Autodesk Inventor part; units mm, degrees
ref_plane "YZ Plane" through (0, 0, 0) normal (1, 0, 0) x (0, 1, 0)
ref_plane "XZ Plane" through (0, 0, 0) normal (0, 1, 0) x (-1, 0, 0)
ref_plane "XY Plane" through (0, 0, 0) normal (0, 0, 1) x (1, 0, 0)
sketch "スケッチ1" plane through (0, 0, 0) normal (0, 0, 1) x (1, 0, 0)
  circle A0 centre (0, 0) radius 12.5
  dimension "d0" = 25
extrude "押し出し1" add sketch "スケッチ1" along normal blind 2.5
sketch "スケッチ2" plane through (0, 0, 2.5) normal (0, 0, 1) x (1, 0, 0)
  line L0 (0, 0) -> (0, 10)
  dimension "d3" = 10
sketch "スケッチ3" plane through (0, 0, 2.5) normal (0, 0, 1) x (1, 0, 0)
  circle A0 centre (0, 9.9998) radius 1
  line L0 (0, 0) -> (0, -10)
  dimension "d4" = 2
  dimension "d5" = 10
sketch "スケッチ4" plane through (0, 0, 2.5) normal (0, 0, 1) x (1, 0, 0)
  circle A0 centre (0, -10) radius 1
  point P0 (0, 0)
  dimension "d6" = 2
sketch "スケッチ5" plane through (0, 0, 2.5) normal (0, 0, 1) x (1, 0, 0)
  line L0 (0, 0) -> (-10, 0)
  dimension "d7" = 10
sketch "スケッチ6" plane through (0, 0, 2.5) normal (0, 0, 1) x (1, 0, 0)
  circle A0 centre (-10.0003, 0) radius 1
  line L0 (0, 0) -> (10, 0)
  circle A1 centre (10, 0) radius 1
  dimension "d8" = 2
  dimension "d9" = 10
  dimension "d10" = 2
extrude "押し出し2" cut sketch "スケッチ3" against normal blind 2.5
extrude "押し出し3" cut sketch "スケッチ6" against normal blind 2.5
extrude "押し出し4" cut sketch "スケッチ4" against normal blind 2.5
sketch "スケッチ7" plane through (0, 0, 2.5) normal (0, 0, 1) x (1, 0, 0)
  line L0 (0, 0) -> (7.0711, 7.0711)
  line L1 (0, 0) -> (10, 0) construction
  line L2 (0, 0) -> (-7.0711, 7.0711)
  line L3 (0, 0) -> (10, 0) construction
  circle A0 centre (-7.0711, 7.0711) radius 1
  circle A1 centre (7.0711, 7.0711) radius 1
  dimension "d17" = 10
  dimension "d18" = 45
  dimension "d19" = 10
  dimension "d20" = 135
  dimension "d21" = 2
  dimension "d22" = 2
sketch "スケッチ8" plane through (0, 0, 2.5) normal (0, 0, 1) x (1, 0, 0)
  line L0 (0, 0) -> (-7.0711, -7.0711)
  line L1 (0, 0) -> (10, 0) construction
  circle A0 centre (-7.0711, -7.0711) radius 1
  line L2 (0, 0) -> (7.0711, -7.0711)
  line L3 (0, 0) -> (10, 0) construction
  circle A1 centre (7.0711, -7.0711) radius 1
  dimension "d23" = 10
  dimension "d24" = 135
  dimension "d25" = 2
  dimension "d26" = 10
  dimension "d27" = 45
  dimension "d28" = 2
extrude "押し出し5" cut sketch "スケッチ7" against normal blind 2.5
extrude "押し出し6" cut sketch "スケッチ8" against normal blind 2.5
sketch "スケッチ9" plane through (0, 0, 2.5) normal (0, 0, 1) x (1, 0, 0)
  point P0 (0, 0)
properties part number "Slit_disk"
The listing builds one solid part. Answer for the finished solid, in the listing's coordinates (mm). Round coordinates to 2 decimals unless told otherwise and drop trailing zeros. Loops run counter-clockwise (first coordinate to the right, second up) from the corner with the lowest first, then second, coordinate; pieces in that order, holes last. Notation, with made-up numbers: (67.25, -6.75) - (101.25, -6.75) arc R26 ccw to (101.25, 21.25) - close; hole circle Ø10 at (14.5, 39.5). An arc over 180 degrees is marked (long way). Return JSON: item names as keys, results as strings. Group by question number.
1. The part is cut by section A-A on x = 10. Determine the outline of the cut face in (y, z).
2. The mould has two halves that part along Y. Classify faces 1 (the cylindrical face through (0, -9, 1)), 2 (the flat face through (0, 0, 0)), 3 (the cylindrical face through (11.923, -3.755, 1.232)): pulls with the +Y half, pulls with the -Y half, needs draft (parallel to the pull), parting line crosses it, or undercut.
3. The part is cut by section C-C on y = 0. Determine the outline of the cut face in (x, z).
4. Consider probe 1 along Y at (x, z) = (6.75, 1.55); probe 2 along Y at (x, z) = (-10.5, 1.05); probe 3 along X at (y, z) = (9.75, 1.9). Determine where each line is inside the solid, lowest interval first.
5. This flat-tipped pin is pushed along its axis until it touches: P1, Ø1.6, axis at x = -7.07, y = -7.07, coming from the -Z side. Where does it stop, or does it pass through?
Resolved:
{
 "1": {"outline": "(-7.5, 0) - (-1, 0) - (-1, 2.5) - (-7.5, 2.5) - close; (1, 0) - (7.5, 0) - (7.5, 2.5) - (1, 2.5) - close"},
 "2": {"face 1": "undercut", "face 2": "needs draft", "face 3": "parting line crosses it"},
 "3": {"outline": "(-12.5, 0) - (-11, 0) - (-11, 2.5) - (-12.5, 2.5) - close; (-9, 0) - (9, 0) - (9, 2.5) - (-9, 2.5) - close; (11, 0) - (12.5, 0) - (12.5, 2.5) - (11, 2.5) - close"},
 "4": {"probe 1": "y = -10.52 to -8.02, -6.12 to 6.12, 8.02 to 10.52", "probe 2": "y = -6.78 to -0.87, 0.87 to 6.78", "probe 3": "x = -7.82 to -0.97, 0.97 to 7.82"},
 "5": {"P1": "passes through"}
}
